Geometry: see drawing. Coordinates: mm, zero at the bounding-box minimum. Give positions to 0.01 mm unless a question says otherwise; leave off trailing zeros. Write each loop counter-clockwise with the first axis right and the second up, starting at its lowest first coordinate (ties: lowest second). Pieces come first, ordered by that corner, then holes. Notation, with made-up numbers: (-36, 25) - (-28, 25) arc R16 cw to (-28, 46) - close; hole circle Ø3 at (-19.75, 75.25). An arc over 180 degrees is marked (long way). Use a Markdown table: item, result. Add a question column.
1. Material intervals for probe 1 along X at (y, z) = (17.5, 69.5) (1 decimal); probe 2 along X at (y, z) = (2, 40) (1 decimal); probe 3 along Y at (x, z) = (12.5, 45) (1 decimal), sorted ascending.
2. Pin query (flat end, axial travel): pin 1 (1 mm diameter, centred on x = 4.5, z = 36.5, fed in from +Y); pin 2 (1.5 mm diameter, centred on x = 18, z = 31.5, fed in from +Y); pin 3 (1 mm diameter, centred on y = 19, z = 51, fed in from -X). Return the tip coordinate at first contact, or that it passes through.
3. Section query C-C, the plane x = 27. Return loops of the section in (y, z).
4. Section query A-A, the plane z = 33. Return loops of the section in (x, y) (1 decimal).
5. Section query B-B, the plane y = 3.5. Return loops of the section in (x, z), plus the area to 3 significant figures.
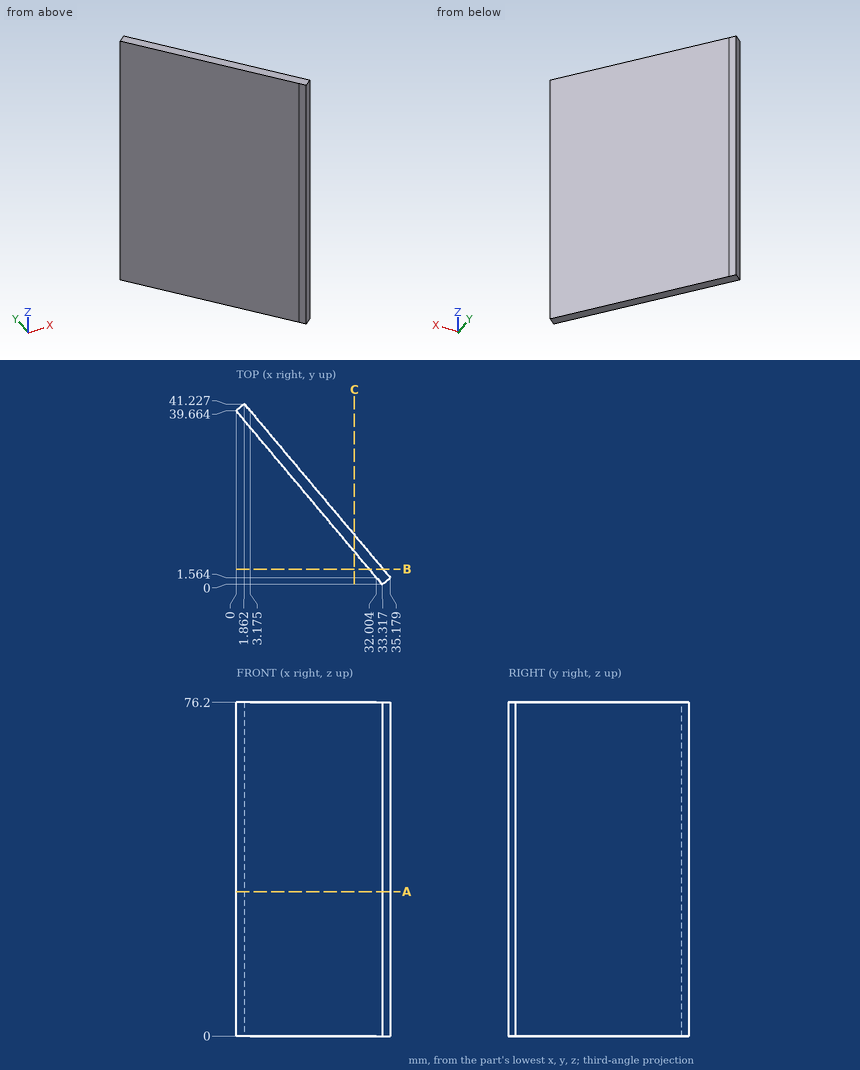
Result sheet:
| question | item | result |
|---|---|---|
| 1 | probe 1 | x = 18.6 to 21.8 |
| 1 | probe 2 | x = 31.6 to 34.8 |
| 1 | probe 3 | y = 24.8 to 28.6 |
| 2 | pin 1 | stops at y = 38.68 |
| 2 | pin 2 | stops at y = 22.91 |
| 2 | pin 3 | stops at x = 16.94 |
| 3 | outline | (7.52, 0) - (11.3, 0) - (11.3, 76.2) - (7.52, 76.2) - close |
| 4 | outline | (0, 39.7) - (33.3, 0) - (35.2, 1.6) - (1.9, 41.2) - close |
| 5 | outline | (30.38, 0) - (33.55, 0) - (33.55, 76.2) - (30.38, 76.2) - close |
| 5 | area | 242 mm² |
